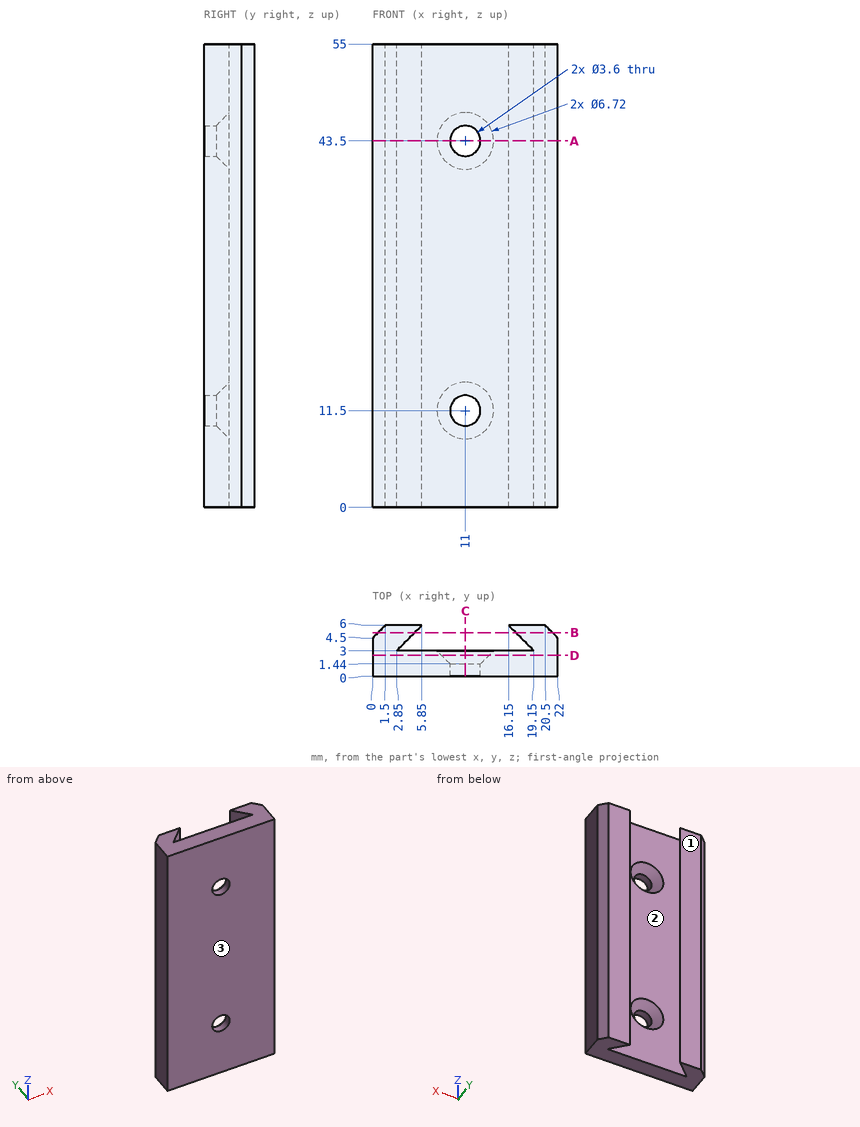
Drawing for the job (mm, zero at the part's lowest x, y, z). Round coordinates to 2 decimals unless told otherwise and drop trailing zeros. Write each loop counter-clockwise with the first axis right and the second up, starting at its lowest first coordinate (ties: lowest second). Pieces come first, ordered by that corner, then holes.
Item 1: Band-saw the part on D-D on y = 2.45. Write the cut outline in (x, z).
Filled in:
outline: (0, 0) - (22, 0) - (22, 55) - (0, 55) - close; hole circle Ø5.62 at (11, 11.5); hole circle Ø5.62 at (11, 43.5)
Item 2: Drop flat-ended pins along their axis: pin 1 Ø5 at (x, z) = (8, 20.5) entering from +Y; pin 2 Ø1 at (x, z) = (7, 44) entering from +Y; pin 3 Ø6 at (x, z) = (11, 11.5) entering from +Y. Give the stop position or say it passes through.
Filled in:
pin 1: stops at y = 6
pin 2: stops at y = 3
pin 3: stops at y = 2.64
Item 3: Band-saw the part on C-C on x = 11. Write the cut outline in (y, z), then the cut area to 3 significant figures.
Filled in:
outline: (0, 0) - (3, 0) - (3, 8.14) - (1.44, 9.7) - (0, 9.7) - close; (0, 13.3) - (1.44, 13.3) - (3, 14.86) - (3, 40.14) - (1.44, 41.7) - (0, 41.7) - close; (0, 45.3) - (1.44, 45.3) - (3, 46.86) - (3, 55) - (0, 55) - close
area: 139 mm2
Item 4: Band-saw the part on A-A on z = 43.5. Write the cut outline in (x, y).
Filled in:
outline: (0, 0) - (9.2, 0) - (9.2, 1.44) - (7.64, 3) - (2.85, 3) - (5.85, 6) - (1.5, 6) - (0, 4.5) - close; (12.8, 0) - (22, 0) - (22, 4.5) - (20.5, 6) - (16.15, 6) - (19.15, 3) - (14.36, 3) - (12.8, 1.44) - close
Item 5: Mould opens along Y. For the marked faces 1, 2 and 3 say: released by +Y, released by -Y, zero draft, split by the parting line, or undercut.
Filled in:
face 1: released by +Y
face 2: undercut
face 3: released by -Y
Item 6: Band-saw the part on B-B on y = 5.15. Write the cut outline in (x, z).
Filled in:
outline: (0.65, 0) - (5, 0) - (5, 55) - (0.65, 55) - close; (17, 0) - (21.35, 0) - (21.35, 55) - (17, 55) - close
Item 7: Drill centre lines: L1, parallel to Z at x = 11, y = 0.9; L2, parallel to X at y = 0.45, z = 43.5; L3, parallel to Z at x = 10, y = 2.45. Where is each one in solid material? Low to high.
Filled in:
L1: z = 0 to 9.7, 13.3 to 41.7, 45.3 to 55
L2: x = 0 to 9.2, 12.8 to 22
L3: z = 0 to 8.87, 14.13 to 40.87, 46.13 to 55
